Autodesk Inventor part; units mm, degrees
ref_plane "YZ Plane" through (0, 0, 0) normal (1, 0, 0) x (0, 1, 0)
ref_plane "XZ Plane" through (0, 0, 0) normal (0, 1, 0) x (-1, 0, 0)
ref_plane "XY Plane" through (0, 0, 0) normal (0, 0, 1) x (1, 0, 0)
sketch "スケッチ1" plane through (0, 0, 0) normal (0, 0, 1) x (1, 0, 0)
  circle A0 centre (0, 0) radius 152
  dimension "d0" = 304
extrude "押し出し1" add sketch "スケッチ1" along normal blind 15
sketch "スケッチ2" plane through (0, 0, 0) normal (0, 0, -1) x (-1, 0, 0)
  point P0 (0, 0)
  point P1 (0, 0)
hole "穴1" at (0, 0, 0) direction (0, 0, 1) diameter 12 end through all
sketch "スケッチ3" plane through (0, 0, 0) normal (0, 0, -1) x (-1, 0, 0)
  circle A0 centre (0, 0) radius 6
sketch "スケッチ4" plane through (0, 0, 15) normal (0, 0, 1) x (1, 0, 0)
  line L0 (-7.8, -2) -> (-2.8778, -2)
  line L1 (-2.8778, -2) -> (-2.8778, 2)
  line L2 (-2.8778, 2) -> (-7.8, 2)
  line L3 (-7.8, 2) -> (-7.8, -2)
  point P0 (0, 0)
  point P1 (-7.8, 0)
  dimension "d10" = 7.8
  dimension "d11" = 2
  dimension "d12" = 2
extrude "押し出し2" cut sketch "スケッチ4" against normal blind 20
properties part number "計測輪"
For this review, take the finished solid that the model builds, in its own axes (mm). Round coordinates to 2 decimals unless told otherwise and drop trailing zeros. Write each loop counter-clockwise with the first axis right and the second up, starting at its lowest first coordinate (ties: lowest second). Pieces come first, ordered by that corner, then holes. Notation, with made-up numbers: (-26, 32.5) -> (-9, 32.5) arc R15 ccw to (-9, 41.5) -> close; hole circle Ø7 at (-19, -3). An arc over 180 degrees is marked (long way). One line per question, with ' | ' between items. Start each with the question number.
1) Add section B-B (z = 10.5). Write out the cut boundary in (x, y), and give its area (3 significant figures).
2) Wall thickness on line 1 along Y through (x, z) = (0, 3.5); line 2 along Y through (x, z) = (-104, 6.5); line 3 along Y through (x, z) = (-78, 11): over which ranges is each line inside the solid? List them lowest first.
3) For pin 1 Ø2.5 at (x, z) = (-7, 10) entering from +Y; pin 2 Ø3 at (y, z) = (-32.5, 13.5) entering from +X; pin 3 Ø7 at (x, y) = (0, 0) entering from -Z; pin 4 Ø2 at (x, z) = (117.5, 2) entering from +Y, all flat-tipped, find the tip position at first contact; note any pin that passes through.
4) Add section D-D (x = -111.5). Write out the cut boundary in (y, z), and give its area (3 significant figures).
5) Add section A-A (x = 0). Write out the cut boundary in (y, z).
6) Mouldability with a two-part tool opening along Y and no side actions: class faces 1 (the cylindrical face through (6, 0, 8)), 2 (the cylindrical face through (70.14, 134.85, 7.4)), 3 (the flat face through (-2, -32, 0)) as +Y half, -Y half, draft (parallel to the pull), parting line (faces both ways), or undercut.
7) Add section C-C (y = 127). Write out the cut boundary in (x, z), and give its area (3 significant figures).
Reported:
1) outline: circle Ø304 at (0, 0); hole (-7.8, -2) -> (-5.66, -2) arc R6 ccw (long way) to (-5.66, 2) -> (-7.8, 2) -> close | area: 72,500 mm²
2) line 1: y = -152 to -6, 6 to 152 | line 2: y = -110.85 to 110.85 | line 3: y = -130.46 to 130.46
3) pin 1: stops at y = 151.89 | pin 2: stops at x = 148.81 | pin 3: passes through | pin 4: stops at y = 97.63
4) outline: (-103.3, 0) -> (103.3, 0) -> (103.3, 15) -> (-103.3, 15) -> close | area: 3,100 mm²
5) outline: (-152, 0) -> (-6, 0) -> (-6, 15) -> (-152, 15) -> close; (6, 0) -> (152, 0) -> (152, 15) -> (6, 15) -> close
6) face 1: undercut | face 2: parting line | face 3: draft
7) outline: (-83.52, 0) -> (83.52, 0) -> (83.52, 15) -> (-83.52, 15) -> close | area: 2,510 mm²
